from build123d import *

# Parameters (mm, degrees)
F1_DEPTH  = 76.2
F2_R      = 10.16
F3_R      = 10.16
F4_DEPTH  = 76.201
F6_DEPTH  = 27.94
F8_DEPTH  = 10.16
F9_R      = 7.62
F10_DEPTH = 25.401


with BuildPart() as f1:
    # F0 (on Front) → F1 (new body)
    with BuildSketch(Plane.XZ):
        Polygon((-35.56, 35.56), (0, 0), (111.76, 0), (111.76, 35.56), (35.56, 35.56), (0, 71.12), (-35.56, 71.12), align=None)
    extrude(amount=F1_DEPTH)

    # F2
    f2_edges = [f1.edges().sort_by_distance(p)[0] for p in [
        (111.76, -76.2, 17.78),
        (111.76, 0, 17.78),
    ]]
    fillet(f2_edges, radius=F2_R)

    # F3 (on Front) → F4 (cut, through all)
    with BuildSketch(Plane.XZ):
        with Locations((17.78, 20.32)):
            Circle(F3_R)
    extrude(amount=F4_DEPTH, mode=Mode.SUBTRACT)

    # F5 (on face) → F6 (cut)
    with BuildSketch(Plane.XY.offset(71.12)):
        with BuildLine():
            ThreePointArc((-10.165424, -15.527446), (-17.636252, -7.621356), (-25.4, -15.24))
            Line((-25.4, -15.24), (-25.4, -60.96))
            ThreePointArc((-25.4, -60.96), (-17.782712, -68.577288), (-10.165424, -60.96))
            Line((-10.165424, -60.96), (-10.165424, -15.527446))
        make_face()
    extrude(amount=-F6_DEPTH, mode=Mode.SUBTRACT)

    # F7 (on face) → F8 (cut)
    with BuildSketch(Plane.XY.offset(35.56)):
        with BuildLine():
            ThreePointArc((93.820625, -40.64), (93.940117, -39.372498), (93.98, -38.1))
            ThreePointArc((93.98, -38.1), (93.940117, -36.827502), (93.820625, -35.56))
            ThreePointArc((93.820625, -35.56), (73.66, -17.78), (53.499375, -35.56))
            ThreePointArc((53.499375, -35.56), (53.34, -38.1), (53.499375, -40.64))
            ThreePointArc((53.499375, -40.64), (73.66, -58.42), (93.820625, -40.64))
        make_face()
        with BuildLine():
            ThreePointArc((93.820625, -35.56), (93.940117, -36.827502), (93.98, -38.1))
            ThreePointArc((93.98, -38.1), (93.940117, -39.372498), (93.820625, -40.64))
            Line((93.820625, -40.64), (111.76, -40.64))
            Line((111.76, -40.64), (111.76, -35.56))
            Line((111.76, -35.56), (93.820625, -35.56))
        make_face()
        with BuildLine():
            ThreePointArc((53.499375, -40.64), (53.34, -38.1), (53.499375, -35.56))
            Line((53.499375, -35.56), (35.56, -35.56))
            Line((35.56, -35.56), (35.56, -40.64))
            Line((35.56, -40.64), (53.499375, -40.64))
        make_face()
    extrude(amount=-F8_DEPTH, mode=Mode.SUBTRACT)

    # F9 (on face) → F10 (cut, through all)
    with BuildSketch(Plane.XY.offset(25.4)):
        with Locations((73.66, -38.1)):
            Circle(F9_R)
    extrude(amount=-F10_DEPTH, mode=Mode.SUBTRACT)


solid = f1.part
Verification items for the finished model (mm, model axes). A direction names the side the tool comes from. Round coordinates to 2 decimals unless told otherwise and drop trailing zeros. Write each loop counter-clockwise with the first axis right and the second up, starting at its lowest first coordinate (ties: lowest second). Pieces come first, ordered by that corner, then holes.
(1) Section check A-A (y = -38.1). Enter the section's corners in (x, z), plus the area to 3 significant figures.
Returned:
outline: (-35.56, 35.56) - (0, 0) - (66.04, 0) - (66.04, 25.4) - (35.56, 25.4) - (35.56, 35.56) - (0, 71.12) - (-10.17, 71.12) - (-10.17, 43.18) - (-25.4, 43.18) - (-25.4, 71.12) - (-35.56, 71.12) - close; (81.28, 0) - (111.76, 0) - (111.76, 25.4) - (81.28, 25.4) - close; hole circle Ø20.32 at (17.78, 20.32)
area: 4,590 mm2
(2) Section check D-D (y = -13.5). Enter the section's corners in (x, z), plus the area to 3 significant figures.
Returned:
outline: (-35.56, 35.56) - (0, 0) - (111.76, 0) - (111.76, 35.56) - (35.56, 35.56) - (0, 71.12) - (-10.36, 71.12) - (-10.36, 43.18) - (-25.2, 43.18) - (-25.2, 71.12) - (-35.56, 71.12) - close; hole circle Ø20.32 at (17.78, 20.32)
area: 5,760 mm2
(3) Section check B-B (x = 17.78). Enter the section's corners in (y, z), plus the area to 3 significant figures.
Returned:
outline: (-76.2, 0) - (0, 0) - (0, 10.16) - (-76.2, 10.16) - close; (-76.2, 30.48) - (0, 30.48) - (0, 53.34) - (-76.2, 53.34) - close
area: 2,520 mm2
(4) Access from +Z, -Z, +X, -X, +Y, -Y to the whole of each face (thin tool, end or side, straight path). Record for faces 4 (the flat face through (103, -40.64, 31)), 5 (the cylindrical face through (-17.95, -68.575, 57.346)), 6 (the flat face through (74, -14, 35.56)).
Returned:
face 4: +Z, +X
face 5: +Z
face 6: +Z, +X, +Y, -Y
(5) Mould release check, pull along X, two halves, no side actions. Record for faces 1 (the cylindrical face through (67.613, -42.737, 12.878)), 2 (the flat face through (-10, -38, 71.12)), 3 (the flat face through (-18, -38, 18)): pulls with the +X half, pulls with the -X half, needs draft (parallel to the pull), parting line crosses it, or undercut.
Returned:
face 1: undercut
face 2: needs draft
face 3: pulls with the -X half
(6) Section check C-C (z = 64). Enter the section's corners in (x, y), plus the area to 3 significant figures.
Returned:
outline: (-35.56, -76.2) - (7.12, -76.2) - (7.12, 0) - (-35.56, 0) - close; hole (-25.4, -60.96) arc R7.62 ccw to (-10.17, -60.96) - (-10.17, -15.53) arc R7.62 ccw (long way) to (-25.4, -15.24) - close
area: 2,370 mm2
(7) Material ranges on line 1 (Y direction, x = 73, z = 10); line 2 (X direction, y = -38, z = 18); line 3 (Z direction, x = 65, y = -63), recorded low to high.
Returned:
line 1: y = -76.2 to -45.69, -30.51 to 0
line 2: x = -18 to 7.89, 27.67 to 66.04, 81.28 to 111.76
line 3: z = 0 to 35.56
(8) Depth check by flat-ended pin: pin 1 Ø11 at (x, z) = (103.5, 28.5) entering from -Y; pin 2 Ø20 at (x, y) = (73.66, -38.1) entering from +Z; pin 3 Ø4.5 at (x, y) = (-19.5, -42) entering from +Z; pin 4 Ø8 at (y, z) = (-33.5, 17) entering from -X. Enter the tip coordinate at first touch or a pass-through.
Returned:
pin 1: stops at y = -76.2
pin 2: stops at z = 25.4
pin 3: stops at z = 43.18
pin 4: stops at x = -21
